from build123d import *

# Parameters (mm, degrees)
BOSS_EXTRUDE1_DEPTH               = 36
FILLET1_R                         = 12
M12X1_25_TAPPED_HOLE1_D           = 10.8
M12X1_25_TAPPED_HOLE1_DEPTH       = 24.505352657
M12X1_25_TAPPED_HOLE1_CSINK_D     = 12.05
M12X1_25_TAPPED_HOLE1_CSINK_ANGLE = 90
M12X1_25_TAPPED_HOLE1_TIP         = 3.244647343


with BuildPart() as part:
    # Sketch1 → Boss-Extrude1 (new, symmetric)
    with BuildSketch(Plane.XY):
        Polygon((-28, 3), (-31, 0), (-60, 0), (-60, 10), (-25, 10), (-25, 13), (25, 13), (25, 10), (60, 10), (60, 0), (31, 0), (28, 3), align=None)
    extrude(amount=BOSS_EXTRUDE1_DEPTH, both=True)

    # Fillet1
    fillet1_edges = [part.edges().sort_by_distance(p)[0] for p in [
        (-60, 5, -36),
        (60, 5, -36),
        (60, 5, 36),
        (-60, 5, 36),
    ]]
    fillet(fillet1_edges, radius=FILLET1_R)

    # M12x1.25 Tapped Hole1
    with Locations(Plane(origin=(0, 10, 0), x_dir=(1, 0, 0), z_dir=(0, 1, 0))):
        with Locations((-48, 24), (-48, -24), (48, -24), (48, 24)):
            CounterSinkHole(M12X1_25_TAPPED_HOLE1_D / 2, M12X1_25_TAPPED_HOLE1_CSINK_D / 2, depth=M12X1_25_TAPPED_HOLE1_DEPTH, counter_sink_angle=M12X1_25_TAPPED_HOLE1_CSINK_ANGLE)
            with Locations((0, 0, -(M12X1_25_TAPPED_HOLE1_DEPTH + M12X1_25_TAPPED_HOLE1_TIP / 2))):  # 118° drill point
                Cone(0, M12X1_25_TAPPED_HOLE1_D / 2, M12X1_25_TAPPED_HOLE1_TIP, mode=Mode.SUBTRACT)


solid = part.part
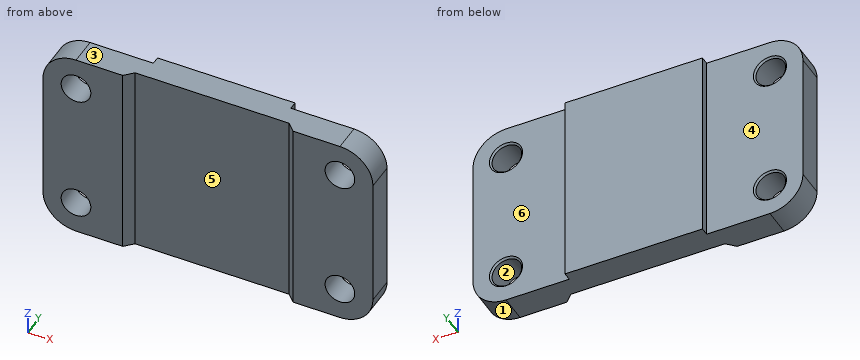
Could you check a few things on this model? Use its own coordinates, in mm. Face numbers are marked on the shaded views. A direction names the side the tool comes from. Give positions to 0.01 mm unless a question says otherwise; leave off trailing zeros. Write each loop counter-clockwise with the first axis right and the second up, starting at its lowest first coordinate (ties: lowest second). Pieces come first, ordered by that corner, then holes. Notation, with made-up numbers: (33, 7.5) -> (87, 7.5) arc R30 cw to (87, 32.5) -> close; hole circle Ø2 at (-21.75, 29.5). An arc over 180 degrees is marked (long way). Write each question's results on one line, items separated by ' | '. Start each with the question number.
Q1. Which directions (+Z, -Z, +X, -X, +Y, -Y) give clear straight access to the entire face, cutting with the end or side of a thin tool? Please do the marked faces 4, 5 and 6.
Q2. Suppose I cut it at A-A, the plane z = 4.5. List the corners of the cut face in (x, y) for me, and give its area (3 significant figures).
Q3. I need wall thicknesses on probe 1 along Z at (x, y) = (48, 7); probe 2 along X at (y, z) = (7.5, 24); probe 3 along Z at (x, y) = (51.5, 3). Which ranges of each line are inside material? Lowest first, please.
Q4. Suppose I cut it at B-B, the plane x = -32.5. List the corners of the cut face in (y, z) for me, and give its area (3 significant figures).
Q5. I'm going to push flat-ended pins straight in: pin 1 Ø9.5 at (x, z) = (48, -24) entering from -Y; pin 2 Ø10.5 at (x, z) = (34, 17.5) entering from +Y; pin 3 Ø0.9 at (y, z) = (11.5, -15) entering from +X. Where does each tip first touch, or does it pass through?
Q6. We'd pull the mould along X, two halves only. Please class the marked faces 1, 2 and 3: +X half, -X half, draft (parallel to the pull), parting line (faces both ways), or undercut.
Outcome:
1) face 4: +Z, -Z, -X, +Y | face 5: +Z, -Z, -Y | face 6: +Z, -Z, +X, +Y
2) outline: (-60, 0) -> (-31, 0) -> (-28, 3) -> (28, 3) -> (31, 0) -> (60, 0) -> (60, 10) -> (25, 10) -> (25, 13) -> (-25, 13) -> (-25, 10) -> (-60, 10) -> close | area: 1,170 mm2
3) probe 1: -36 to -29.4, -18.6 to 18.6, 29.4 to 36 | probe 2: -60 to -53.4, -42.6 to 42.6, 53.4 to 60 | probe 3: -35.48 to -28.11, -19.89 to 19.89, 28.11 to 35.48
4) outline: (0, -36) -> (10, -36) -> (10, 36) -> (0, 36) -> close | area: 720 mm2
5) pin 1: through | pin 2: y = 10 | pin 3: x = 25
6) face 1: +X half | face 2: undercut | face 3: draft
